Geometry check sheet. Reference: the model listing, model coordinates, mm. A direction names the side the tool comes from. Round coordinates to 2 decimals unless told otherwise and drop trailing zeros. Order: outer loops, then holes, each group sorted by start corner. A loop starts at its lowest first (then second) coordinate and runs counter-clockwise, first axis right, second up.
Autodesk Inventor part; units mm, degrees
ref_plane "YZ Plane" through (0, 0, 0) normal (1, 0, 0) x (0, 1, 0)
ref_plane "XZ Plane" through (0, 0, 0) normal (0, 1, 0) x (-1, 0, 0)
ref_plane "XY Plane" through (0, 0, 0) normal (0, 0, 1) x (1, 0, 0)
sketch "Sketch1" plane through (0, 0, 0) normal (0, 0, 1) x (1, 0, 0)
  line L0 (-241.5, 190.5) -> (241.5, 190.5)
  line L1 (241.5, 190.5) -> (241.5, -190.5)
  line L2 (241.5, -190.5) -> (-241.5, -190.5)
  line L3 (-241.5, -190.5) -> (-241.5, 190.5)
  point P0 (0, 0)
  point P1 (241.5, 0)
  point P2 (0, 190.5)
  dimension "d0" = 483
  dimension "d1" = 381
extrude "Extrusion1" add sketch "Sketch1" along normal blind 43.2
fillet "Fillet1" radius 12.7 4 edges at (241.5, 190.5, 21.6) (-241.5, 190.5, 21.6) (241.5, -190.5, 21.6) (-241.5, -190.5, 21.6)
sketch "Sketch2" plane through (0, 0, 43.2) normal (0, 0, 1) x (1, 0, 0)
  circle A0 centre (0, 0) radius 177.5 construction
  line L0 (-225, 124) -> (-225, -124)
  line L1 (-225, 124) -> (-127.0049, 124)
  line L2 (-241.5, -177.8) -> (-241.5, 177.8)
  line L3 (-225, -124) -> (-127.0049, -124)
  arc A1 (-127.0049, -124) -> (-127.0049, 124) centre (0, 0) ccw
  point P0 (-225, 0)
  dimension "d5" = 355
  dimension "d6" = 248
  dimension "d7" = 225
extrude "Extrusion2" add sketch "Sketch2" along normal blind 286.8
sketch "Sketch3" plane through (-225, -124, 43.2) normal (-1, 0, 0) x (0, 0, 1)
  line L0 (191.2, 243) -> (74.2, 243)
  line L1 (74.2, 243) -> (74.2, 5)
  line L2 (74.2, 5) -> (191.2, 5)
  line L3 (191.2, 5) -> (191.2, 243)
  line L4 (0, 301.8) -> (0, -53.8)
  point P0 (-43.2, 124)
  point P1 (191.2, 124)
  point P2 (0, 124)
  dimension "d10" = 238
  dimension "d11" = 117
  dimension "d12" = 74.2
extrude "Extrusion3" add sketch "Sketch3" along normal blind 51
sketch "Sketch4" plane through (0, 0, 330) normal (0, 0, 1) x (1, 0, 0)
  circle A0 centre (0, 0) radius 125 construction
  circle A1 centre (-150, 0) radius 48.5 construction
  line L0 (-150, 48.5) -> (-115.2074, 48.5)
  line L1 (-150, -48.5) -> (-115.2074, -48.5)
  arc A2 (-150, 48.5) -> (-150, -48.5) centre (-150, 0) ccw
  arc A3 (-115.2074, -48.5) -> (-115.2074, 48.5) centre (0, 0) ccw
  dimension "d15" = 250
  dimension "d16" = 97
  dimension "d17" = 150
extrude "Extrusion4" add sketch "Sketch4" along normal blind 19
sketch "Sketch5" plane through (0, 0, 349) normal (0, 0, 1) x (1, 0, 0)
  arc A0 (-150, 48.5) -> (-150, -48.5) centre (-150, 0) ccw
  circle A1 centre (-150, 0) radius 48.5
  point P0 (0, 0)
extrude "Extrusion5" add sketch "Sketch5" along normal blind 64
sketch "Sketch6" plane through (0, 0, 349) normal (0, 0, 1) x (1, 0, 0)
  circle A0 centre (0, 0) radius 84
  dimension "d22" = 168
extrude "Extrusion6" add sketch "Sketch6" along normal blind 479
properties part number "Base"
(1) Sectioned sample at B-B, the plane x = 0. Record the cut outline in (y, z).
Returned:
outline: (-190.5, 0) - (190.5, 0) - (190.5, 43.2) - (177.5, 43.2) - (177.5, 330) - (125, 330) - (125, 349) - (84, 349) - (84, 828) - (-84, 828) - (-84, 349) - (-125, 349) - (-125, 330) - (-177.5, 330) - (-177.5, 43.2) - (-190.5, 43.2) - close
(2) Set-up check for faces 1 (the flat face through (-177, -124, 185)), 2 (the flat face through (-133, 48.5, 339)), 3 (the flat face through (-1, 1, 828)), 4 (the flat face through (16, 85, 349)), 5 (the flat face through (-151, 1, 413)): record each of +Z, -Z, +X, -X, +Y, -Y from which the full face is reachable in a straight line by a thin tool's end or side.
Returned:
face 1: +Z, -X, -Y
face 2: +Z, -X, +Y
face 3: +Z, +X, -X, +Y, -Y
face 4: +Z
face 5: +Z, -X, +Y, -Y
(3) Sectioned sample at C-C, the plane y = -155. Record the cut outline in (x, z), and give its area (3 significant figures).
Returned:
outline: (-241.5, 0) - (241.5, 0) - (241.5, 43.2) - (86.49, 43.2) - (86.49, 330) - (-86.49, 330) - (-86.49, 43.2) - (-241.5, 43.2) - close
area: 70,500 mm2
(4) Draft check along Z on faces 6 (the flat face through (-177, 124, 185)), 7 (the flat face through (-250, -2, 234.4)), 8 (the flat face through (-3, 3, 0)), 9 (the flat face through (-225, 2, 248)). Enter one of: released by +Z, released by -Z, zero draft, split by the parting line, or undercut.
Returned:
face 6: zero draft
face 7: released by +Z
face 8: released by -Z
face 9: undercut
(5) Depth check by flat-ended pin: P1, Ø1.5, axis at x = 40.5, z = 236, coming from the +Y side; P2, Ø8, axis at y = 10, z = 230, coming from the +X side; P3, Ø15, axis at x = -126.5, z = 341, coming from the +Y side. Enter the tip coordinate at first touch or a pass-through.
Returned:
P1: stops at y = 172.99
P2: stops at x = 177.4
P3: stops at y = 48.5
(6) Material ranges on line 1 (Z direction, x = -32, y = -161.5); line 2 (Y direction, x = -4.5, z = 601); line 3 (Z direction, x = -192, y = -153), recorded low to high.
Returned:
line 1: z = 0 to 330
line 2: y = -83.88 to 83.88
line 3: z = 0 to 43.2
(7) Sectioned sample at D-D, the plane x = 96. Record the cut outline in (y, z).
Returned:
outline: (-190.5, 0) - (190.5, 0) - (190.5, 43.2) - (149.3, 43.2) - (149.3, 330) - (80.06, 330) - (80.06, 349) - (-80.06, 349) - (-80.06, 330) - (-149.3, 330) - (-149.3, 43.2) - (-190.5, 43.2) - close
(8) Sectioned sample at A-A, the plane z = 361. Record the cut outline in (x, y), and give its area (3 significant figures).
Returned:
outline: circle Ø97 at (-150, 0); circle Ø168 at (0, 0)
area: 29,600 mm2
